from build123d import *

# Parameters (mm, degrees)
BOSS_EXTRU_1_DEPTH      = 60
ESQUISSE2_R             = 30
ESQUISSE2_R_2           = 29
BOSS_EXTRU_2_DEPTH      = 60
ESQUISSE3_R             = 25
ENL_V_MAT_EXTRU_1_DEPTH = 27
ESQUISSE6_R             = 2.225
ENL_V_MAT_EXTRU_3_DEPTH = 2
ESQUISSE11_R            = 25
ESQUISSE11_R_2          = 3.5
ENL_V_MAT_EXTRU_8_DEPTH = 31


with BuildPart() as part:
    # Esquisse1 → Boss.-Extru.1 (new body)
    with BuildSketch(Plane.XY):
        with BuildLine():
            Line((1, -15.006468588), (1, -3.354101966))
            ThreePointArc((1, -3.354101966), (3.5, 0), (1, 3.354101966))
            Line((1, 3.354101966), (1, 29.5))
            Line((1, 29.5), (-1, 29.5))
            Line((-1, 29.5), (-1, 3.354101966))
            ThreePointArc((-1, 3.354101966), (-3.5, 0), (-1, -3.354101966))
            Line((-1, -3.354101966), (-1, -29.5))
            Line((-1, -29.5), (1, -29.5))
            Line((1, -29.5), (1, -15.006468588))
        make_face()
    extrude(amount=BOSS_EXTRU_1_DEPTH)

    # Esquisse2 → Boss.-Extru.2 (add)
    with BuildSketch(Plane.XY.offset(60)):
        Circle(ESQUISSE2_R)
        Circle(ESQUISSE2_R_2, mode=Mode.SUBTRACT)
    extrude(amount=-BOSS_EXTRU_2_DEPTH)

    # Esquisse3 → Enlèv. mat.-Extru.1 (cut)
    with BuildSketch(Plane.XY.offset(60)):
        Circle(ESQUISSE3_R)
    extrude(amount=-ENL_V_MAT_EXTRU_1_DEPTH, mode=Mode.SUBTRACT)

    # Esquisse6 → Enlèv. mat.-Extru.3 (cut)
    with BuildSketch(Plane.XY.offset(33)):
        Circle(ESQUISSE6_R)
    extrude(amount=-ENL_V_MAT_EXTRU_3_DEPTH, mode=Mode.SUBTRACT)

    # Esquisse11 → Enlèv. mat.-Extru.8 (cut)
    with BuildSketch(Plane.XY.offset(60)):
        Circle(ESQUISSE11_R)
        Circle(ESQUISSE11_R_2, mode=Mode.SUBTRACT)
    extrude(amount=-ENL_V_MAT_EXTRU_8_DEPTH, mode=Mode.SUBTRACT)


solid = part.part
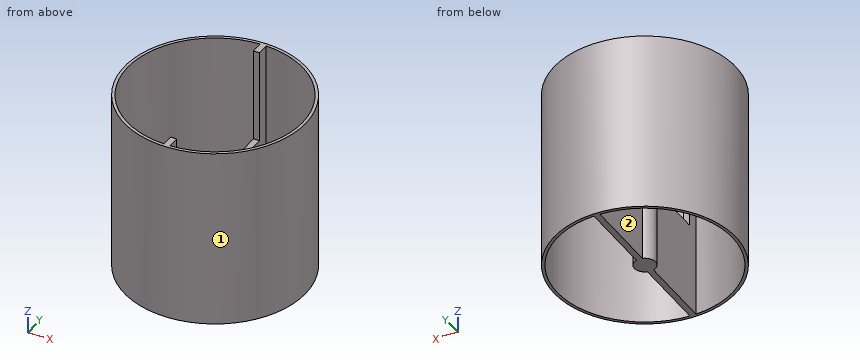
Could you check a few things on this model? Use its own coordinates, in mm. Face numbers are marked on the shaded views. Give positions to 0.01 mm unless a question says otherwise; leave off trailing zeros. Order: outer loops, then holes, each group sorted by start corner. A loop starts at its lowest first (then second) coordinate and runs counter-clockwise, first axis right, second up.
Item 1: I'm going to push flat-ended pins straight in: pin 1 (3.5 mm diameter, centred on x = -1, y = 1.5, fed in from +Z); pin 2 (3.5 mm diameter, centred on x = 0, y = 0, fed in from +Z); pin 3 (4 mm diameter, centred on y = -9.5, z = 21.5, fed in from -X). Where does each tip first touch, or does it pass through?
Item 2: If we mould it in two halves opening along X, with no side actions, what happens to the marked faces 1 and 2? For each: pulls with the +X half, pulls with the -X half, needs draft (parallel to the pull), parting line crosses it, or undercut.
Item 3: If we section it at C-C, the plane x = 13: Write out the boundary of the cut face in (y, z).
Item 4: I need wall thicknesses on line 1 (Y direction, x = 0, z = 31.55) (3 decimals); line 2 (X direction, y = 22.5, z = 27); line 3 (Y direction, x = 0, z = 57). Which ranges of each line are inside material? Lowest first, please.
Item 5: If we section it at B-B, the plane z = 32: Write out the boundary of the cut face in (x, y) (3 decimals).
Item 6: If we section it at A-A, the plane y = 0: Write out the boundary of the cut face in (x, z) (3 decimals), plus the area to 3 significant figures.
Values:
1. pin 1: stops at z = 33
1. pin 2: stops at z = 31
1. pin 3: stops at x = -29.05
2. face 1: parting line crosses it
2. face 2: undercut
3. outline: (-27.04, 0) - (-25.92, 0) - (-25.92, 60) - (-27.04, 60) - close; (25.92, 0) - (27.04, 0) - (27.04, 60) - (25.92, 60) - close
4. line 1: y = -30 to -25, -3.5 to -2.225, 2.225 to 3.5, 25 to 30
4. line 2: x = -19.84 to -18.3, -1 to 1, 18.3 to 19.84
4. line 3: y = -30 to -25, 25 to 30
5. outline: circle Ø60 at (0, 0); circle Ø7 at (0, 0); hole circle Ø4.45 at (0, 0); hole (-1, -28.983) - (-1, -24.98) arc R25 ccw to (1, -24.98) - (1, -28.983) arc R29 ccw to (1, 28.983) - (1, 24.98) arc R25 ccw to (-1, 24.98) - (-1, 28.983) arc R29 ccw to start
6. outline: (-30, 0) - (-29, 0) - (-29, 60) - (-30, 60) - close; (-3.5, 0) - (3.5, 0) - (3.5, 33) - (2.225, 33) - (2.225, 31) - (-2.225, 31) - (-2.225, 33) - (-3.5, 33) - close; (29, 0) - (30, 0) - (30, 60) - (29, 60) - close
6. area: 342 mm2
